CAD build for the part. Positions are in the model's coordinates, mm. A direction names the side the tool comes from. Coordinates: 2 decimals unless noted, no trailing zeros. Order: outer loops, then holes, each group sorted by start corner. A loop starts at its lowest first (then second) coordinate and runs counter-clockwise, first axis right, second up. Notation, with made-up numbers: M 77,84 L 110,84 A28 cw 110,112 Z; hole C 24,-24 d8. An arc over 180 degrees is marked long. One line per item, written item: value.
from build123d import *

# Parameters (mm, degrees)
SKETCH1_W      = 18
SKETCH1_H      = 32
EXTRUDE1_DEPTH = 5
SKETCH3_R      = 0.75
SKETCH3_R_2    = 1.4732
EXTRUDE2_DEPTH = 6
SKETCH4_R      = 0.75
EXTRUDE3_DEPTH = 2.794


with BuildPart() as part:
    # Sketch1 → Extrude1 (new body)
    with BuildSketch(Plane.XY):
        with Locations((-9, 16)):
            Rectangle(SKETCH1_W, SKETCH1_H)
    extrude(amount=EXTRUDE1_DEPTH)

    # Sketch2 → #4-40 Tapped Hole1 (revolve, cut)
    with BuildSketch(Plane(origin=(-14, 32, 2.5), x_dir=(0, 0, 1), z_dir=(1, 0, 0))):
        Polygon((0, 0), (0, 10.813752758), (1.1303, 10.1346), (1.1303, 8.2296), (1.4224, 8.2296), (1.4224, 0), align=None)
    f_4_40_tapped_hole1 = revolve(axis=Axis((-14, 38.35, 2.5), (0, -1, 0)), mode=Mode.SUBTRACT)

    # Sketch3 → Extrude2 (cut, through all)
    with BuildSketch(Plane.XY.offset(5)):
        with Locations((-14, 22)):
            Circle(SKETCH3_R)
        with Locations((-14, 2.5)):
            Circle(SKETCH3_R_2)
    extrude2 = extrude(amount=-EXTRUDE2_DEPTH, mode=Mode.SUBTRACT)

    # Sketch4 → Extrude3 (cut)
    with BuildSketch(Plane.ZY.offset(18)):
        with Locations((2.5, 2.5)):
            Circle(SKETCH4_R)
    extrude3 = extrude(amount=-EXTRUDE3_DEPTH, mode=Mode.SUBTRACT)

    # Mirror2: #4-40 Tapped Hole1, Extrude2, Extrude3 across plane
    add(f_4_40_tapped_hole1.mirror(Plane(origin=(-9, 0, 0), x_dir=(0, 0, 1), z_dir=(1, 0, 0))), mode=Mode.SUBTRACT)
    add(extrude2.mirror(Plane(origin=(-9, 0, 0), x_dir=(0, 0, 1), z_dir=(1, 0, 0))), mode=Mode.SUBTRACT)
    add(extrude3.mirror(Plane(origin=(-9, 0, 0), x_dir=(0, 0, 1), z_dir=(1, 0, 0))), mode=Mode.SUBTRACT)


solid = part.part
Q1. Slice it at A-A (y = 2.5). List the corners of the cut face in (x, z), plus the area to 3 significant figures.
Recorded:
outline: M -18,0 L -15.47,0 L -15.47,1.75 L -18,1.75 Z; M -18,3.25 L -15.47,3.25 L -15.47,5 L -18,5 Z; M -12.53,0 L -5.47,0 L -5.47,5 L -12.53,5 Z; M -2.53,0 L 0,0 L 0,1.75 L -2.53,1.75 Z; M -2.53,3.25 L 0,3.25 L 0,5 L -2.53,5 Z
area: 53.0 mm^2
Q2. Drill centre lines: line 1 along Y through (x, z) = (-14, 4.1); line 2 along X through (y, z) = (23, 2.5); line 3 along X through (y, z) = (2.5, 1.05). Where is each one in solid material? Low to high.
Recorded:
line 1: y = 0 to 1.03, 3.97 to 21.25, 22.75 to 32
line 2: x = -18 to -15.13, -12.87 to -5.13, -2.87 to 0
line 3: x = -18 to -15.47, -12.53 to -5.47, -2.53 to 0
Q3. Mould opens along Z. For faces 4 (the face through (-9, 16, 0)), 5 (the face through (-1.35, 2.53, 1.75)), 6 (the face through (0, 16, 2)) say: released by +Z, released by -Z, zero draft, split by the parting line, or undercut.
Recorded:
face 4: released by -Z
face 5: undercut
face 6: zero draft
Q4. Pin check, flat tip, straight feed: pin 1 Ø3 at (x, z) = (-14.5, 2.5) entering from +Y. Stop position of the tip, or through.
Recorded:
pin 1: stops at y = 32
Q5. Which spindle directions (+Z, -Z, +X, -X, +Y, -Y) get a long thin tool onto all of the face, cutting with end or side? Do faces 1 (the face through (-16.65, 2.53, 1.75)), 2 (the face through (-12.61, 27.94, 2.19)), 3 (the face through (-9, 32, 2)). Say none if no direction does.
Recorded:
face 1: -X
face 2: +Y
face 3: +Z, -Z, +X, -X, +Y
